```python
from build123d import *

# Parameters (mm, degrees)
SKETCH1_R           = 9.65
SKETCH1_R_2         = 4.15
BOSS_EXTRUDE1_DEPTH = 2


with BuildPart() as part:
    # Sketch1 → Boss-Extrude1 (new body)
    with BuildSketch(Plane.XY):
        with BuildLine():
            Line((17.005, -29), (-17.005, -29))
            ThreePointArc((-17.005, -29), (-19.126320344, -28.121320344), (-20.005, -26))
            Line((-20.005, -26), (-20.005, 26))
            ThreePointArc((-20.005, 26), (-19.126320344, 28.121320344), (-17.005, 29))
            Line((-17.005, 29), (17.005, 29))
            ThreePointArc((17.005, 29), (19.126320344, 28.121320344), (20.005, 26))
            Line((20.005, 26), (20.005, -26))
            ThreePointArc((20.005, -26), (19.126320344, -28.121320344), (17.005, -29))
        make_face()
        with Locations((0, 6)):
            Circle(SKETCH1_R, mode=Mode.SUBTRACT)
        with Locations((13.65, 20.15)):
            Circle(SKETCH1_R_2, mode=Mode.SUBTRACT)
        with Locations((6.45, -6.7)):
            Circle(SKETCH1_R_2, mode=Mode.SUBTRACT)
        with Locations((-6.45, -6.7)):
            Circle(SKETCH1_R_2, mode=Mode.SUBTRACT)
        with Locations((-13.65, -20.2)):
            Circle(SKETCH1_R_2, mode=Mode.SUBTRACT)
        with Locations((-13.65, 20.15)):
            Circle(SKETCH1_R_2, mode=Mode.SUBTRACT)
        with BuildLine():
            Line((10.715506858, -23.134493142), (6.472866171, -18.891852455))
            ThreePointArc((6.472866171, -18.891852455), (6.472866171, -13.022866171), (12.341852455, -13.022866171))
            Line((12.341852455, -13.022866171), (16.584493142, -17.265506858))
            ThreePointArc((16.584493142, -17.265506858), (16.584493142, -23.134493142), (10.715506858, -23.134493142))
        make_face(mode=Mode.SUBTRACT)
    extrude(amount=BOSS_EXTRUDE1_DEPTH)


solid = part.part
```
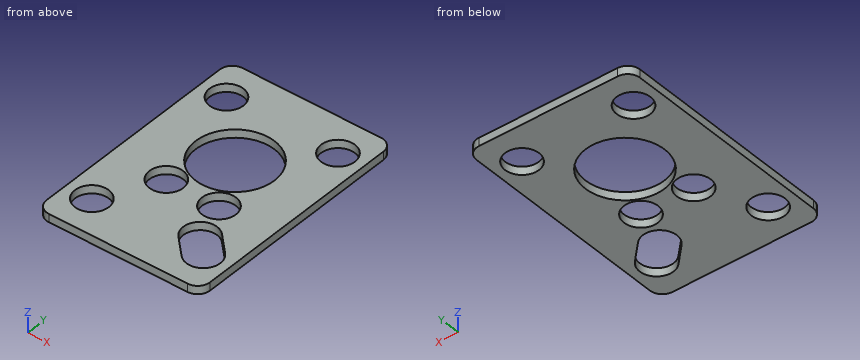
The model under review builds one solid part; all positions refer to its coordinate system, in mm. Round coordinates to 2 decimals unless told otherwise and drop trailing zeros. Loops run counter-clockwise (first coordinate to the right, second up) from the corner with the lowest first, then second, coordinate; pieces in that order, holes last.
Item 1: For line 1 (Y direction, x = -13.65, z = 0.55); line 2 (Y direction, x = -3.5, z = 1); line 3 (Y direction, x = 0, z = 1.5), list the stretches that pass through material, from the lowest coordinate up.
Determined:
line 1: y = -29 to -24.35, -16.05 to 16, 24.3 to 29
line 2: y = -29 to -9.62, -3.78 to -2.99, 14.99 to 29
line 3: y = -29 to -3.65, 15.65 to 29
Item 2: Take a section at C-C (z = 1.2). Give the number of separate pieces and of enclosed holes in the cut face, then the cut area to 3 significant figures.
Determined:
separate pieces: 1
enclosed holes: 7
area: 1,650 mm2
Item 3: Take a section at A-A (x = 0). Write out the cut boundary in (y, z), then the cut area to 3 significant figures.
Determined:
outline: (-29, 0) - (-3.65, 0) - (-3.65, 2) - (-29, 2) - close; (15.65, 0) - (29, 0) - (29, 2) - (15.65, 2) - close
area: 77.4 mm2
Item 4: Take a section at D-D (y = -6.7). Write out the cut boundary in (x, z) (3 decimals).
Determined:
outline: (-20.005, 0) - (-10.6, 0) - (-10.6, 2) - (-20.005, 2) - close; (-2.3, 0) - (2.3, 0) - (2.3, 2) - (-2.3, 2) - close; (10.6, 0) - (20.005, 0) - (20.005, 2) - (10.6, 2) - close
Item 5: Take a section at B-B (y = 6). Write out the cut boundary in (x, z) (3 decimals).
Determined:
outline: (-20.005, 0) - (-9.65, 0) - (-9.65, 2) - (-20.005, 2) - close; (9.65, 0) - (20.005, 0) - (20.005, 2) - (9.65, 2) - close
